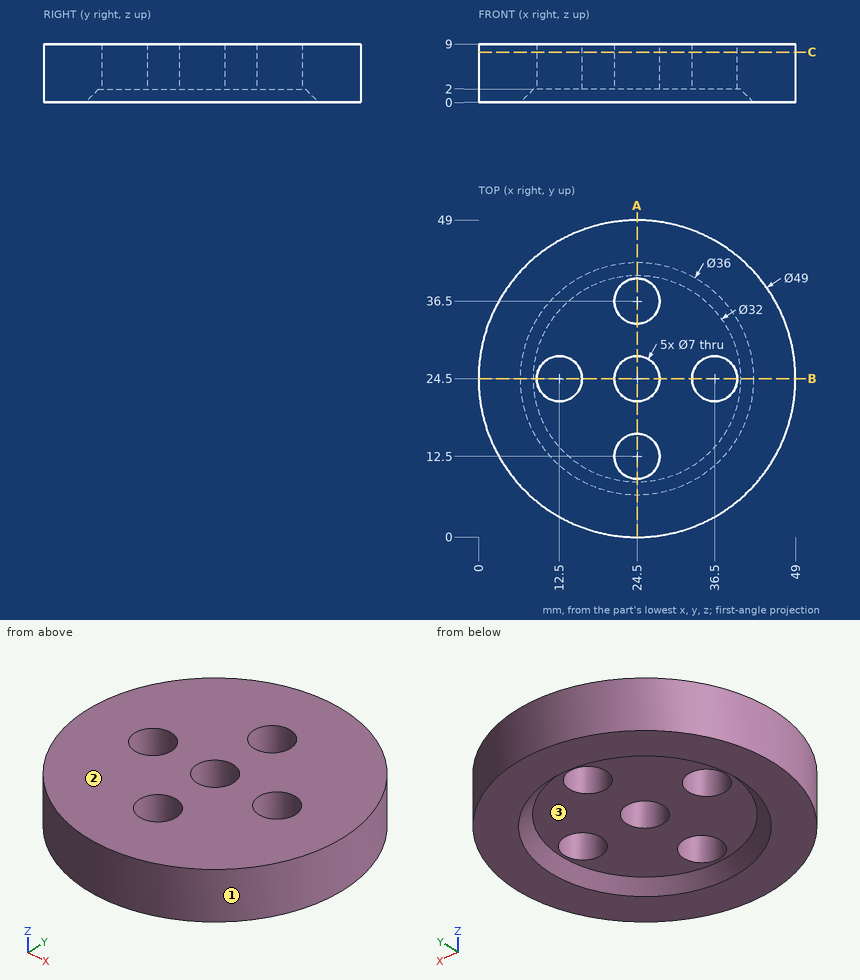
Study the drawing (mm; zero at the part's minimum x, y, z) and answer. Coordinates: 2 decimals unless noted, no trailing zeros. Loops run counter-clockwise (first coordinate to the right, second up) from the corner with the lowest first, then second, coordinate; pieces in that order, holes last. Notation, with made-up numbers: M 30.5,86.25 L 70.5,86.25 A13 ccw 70.5,105.25 Z; hole C 58,41 d3. An arc over 180 degrees is marked long. Answer in a Markdown table with one row per item. Add a question column.
1. The mould has two halves that part along X. Classify the marked faces 1, 2 and 3: pulls with the +X half, pulls with the -X half, needs draft (parallel to the pull), parting line crosses it, or undercut.
2. Find section A-A, the plane x = 24.5. Write down the section's boundary in (y, z).
3. Find section C-C, the plane z = 7.75. Write down the section's boundary in (x, y), then the cut area to 3 significant figures.
4. Flat-ended cylindrical pins translate along their axes: P1, Ø5, axis at y = 12.5, z = 5, coming from the -X side; P2, Ø4, axis at x = 39, z = 3.5, coming from the -Y side; P3, Ø11, axis at x = 24.5, y = 24.5, coming from the -Z side. Find the tip coordinate at first contact, or state that the pin passes through.
5. Consider L1, parallel to Y at x = 24.5, z = 3.75; L2, parallel to X at y = 27.5, z = 8; L3, parallel to Z at x = 19.5, y = 36. Determine where each line is inside the solid, lowest interval first.
Reported:
| question | item | result |
|---|---|---|
| 1 | face 1 | parting line crosses it |
| 1 | face 2 | needs draft |
| 1 | face 3 | undercut |
| 2 | outline | M 0,0 L 6.5,0 L 8.5,2 L 9,2 L 9,9 L 0,9 Z; M 16,2 L 21,2 L 21,9 L 16,9 Z; M 28,2 L 33,2 L 33,9 L 28,9 Z; M 40,2 L 40.5,2 L 42.5,0 L 49,0 L 49,9 L 40,9 Z |
| 3 | outline | C 24.5,24.5 d49; hole C 12.5,24.5 d7; hole C 24.5,12.5 d7; hole C 24.5,24.5 d7; hole C 24.5,36.5 d7; hole C 36.5,24.5 d7 |
| 3 | area | 1,690 mm^2 |
| 4 | P1 | stops at x = 1.92 |
| 4 | P2 | stops at y = 3.43 |
| 4 | P3 | stops at z = 2 |
| 5 | L1 | y = 0 to 9, 16 to 21, 28 to 33, 40 to 49 |
| 5 | L2 | x = 0.18 to 10.7, 14.3 to 22.7, 26.3 to 34.7, 38.3 to 48.82 |
| 5 | L3 | z = 2 to 9 |
